```python
from build123d import *

# Parameters (mm, degrees)
F0_R      = 2
F1_DEPTH  = 6
F3_DEPTH  = 6.001
F5_DEPTH  = 6.001
F6_R      = 5
F7_DEPTH  = 6.001
F8_DEPTH  = 585
F9_R      = 2
F10_DEPTH = 6.001
F12_DEPTH = 2.5
F13_R     = 2


# Not quite as in the source:
# - an extrude ends at something that could not be found from the text; its depth is read off the source's solid


with BuildPart() as f1:
    # F0 (on Front) → F1 (new body)
    with BuildSketch(Plane.XZ):
        with BuildLine():
            Line((61.1081310213, 8.0650188029), (-54.7722764313, 8.0650188029))
            ThreePointArc((-54.7722764313, 8.0650188029), (-58.9525619371, 3.7295520634), (-59.8848706484, -2.2203940898))
            Line((-59.8848706484, -2.2203940898), (-59.8848706484, -29.6689261496))
            ThreePointArc((-59.8848706484, -29.6689261496), (-58.4204045543, -33.2044600555), (-54.8848706484, -34.6689261496))
            Line((-54.8848706484, -34.6689261496), (-38.6363018323, -34.6689261496))
            Line((-38.6363018323, -34.6689261496), (39.8797094822, -34.6689261496))
            Line((39.8797094822, -34.6689261496), (177.1196573973, -60.5151057243))
            Line((177.1196573973, -60.5151057243), (247.381187493, -88.5924363301))
            Line((247.381187493, -88.5924363301), (248.0585300922, -163.5853774846))
            Line((248.0585300922, -163.5853774846), (308.0585300922, -163.5853774846))
            Line((308.0585300922, -163.5853774846), (308.0585300922, -13.5853774846))
            Line((308.0585300922, -13.5853774846), (61.1081310213, 8.0650188029))
        make_face()
        with Locations((35.7915443742, -3.0683759738)):
            Circle(F0_R, mode=Mode.SUBTRACT)
    extrude(amount=F1_DEPTH)

    # F2 (on face) → F3 (cut, through all)
    with BuildSketch(Plane.XZ.offset(6)):
        with BuildLine():
            ThreePointArc((92.5020176823, -9.2679053605), (88.9664837764, -17.8034392664), (97.5020176823, -14.2679053605))
            ThreePointArc((97.5020176823, -14.2679053605), (96.0375515883, -10.7323714546), (92.5020176823, -9.2679053605))
        make_face()
    extrude(amount=-F3_DEPTH, mode=Mode.SUBTRACT)

    # F4 (on face) → F5 (cut, through all)
    with BuildSketch(Plane.XZ.offset(6)):
        with BuildLine():
            ThreePointArc((284.0794362254, -115.9942394993), (281.9581158818, -121.1155598429), (287.0794362254, -118.9942394993))
            ThreePointArc((287.0794362254, -118.9942394993), (286.2007565689, -116.8729191558), (284.0794362254, -115.9942394993))
        make_face()
        with BuildLine():
            ThreePointArc((287.0794362254, -56.0820794532), (281.9581158818, -53.9607591097), (284.0794362254, -59.0820794532))
            ThreePointArc((284.0794362254, -59.0820794532), (286.2007565689, -58.2033997968), (287.0794362254, -56.0820794532))
        make_face()
    extrude(amount=-F5_DEPTH, mode=Mode.SUBTRACT)

    # F6 (on face) → F7 (cut, through all)
    with BuildSketch(Plane(origin=(0, 0, 0), x_dir=(-1, 0, 0), z_dir=(0, 1, 0))):
        with Locations((7.8367077125, 0)):
            Circle(F6_R)
    extrude(amount=-F7_DEPTH, mode=Mode.SUBTRACT)

    # F0 (on Front) → F8 (cut, through all)
    with BuildSketch(Plane.XZ):
        with BuildLine():
            Line((61.1081310213, 8.0650188029), (-54.7722764313, 8.0650188029))
            ThreePointArc((-54.7722764313, 8.0650188029), (-58.9525619371, 3.7295520634), (-59.8848706484, -2.2203940898))
            Line((-59.8848706484, -2.2203940898), (-59.8848706484, -29.6689261496))
            ThreePointArc((-59.8848706484, -29.6689261496), (-58.4204045543, -33.2044600555), (-54.8848706484, -34.6689261496))
            Line((-54.8848706484, -34.6689261496), (-38.6363018323, -34.6689261496))
            Line((-38.6363018323, -34.6689261496), (39.8797094822, -34.6689261496))
            Line((39.8797094822, -34.6689261496), (177.1196573973, -60.5151057243))
            Line((177.1196573973, -60.5151057243), (247.381187493, -88.5924363301))
            Line((247.381187493, -88.5924363301), (248.0585300922, -163.5853774846))
            Line((248.0585300922, -163.5853774846), (308.0585300922, -163.5853774846))
            Line((308.0585300922, -163.5853774846), (308.0585300922, -13.5853774846))
            Line((308.0585300922, -13.5853774846), (61.1081310213, 8.0650188029))
        make_face()
        with Locations((35.7915443742, -3.0683759738)):
            Circle(F0_R, mode=Mode.SUBTRACT)
    extrude(amount=-F8_DEPTH, mode=Mode.SUBTRACT)

    # F9 (on face) → F10 (cut, through all)
    with BuildSketch(Plane.XZ.offset(6)):
        with Locations((144.0575271969, -19.352506299)):
            Circle(F9_R)
    extrude(amount=-F10_DEPTH, mode=Mode.SUBTRACT)

    # F11 (on face) → F12 (cut)
    with BuildSketch(Plane(origin=(0, 0, 0), x_dir=(-1, 0, 0), z_dir=(0, 1, 0))):
        Polygon((-95.3768665934, -0.9623710934), (-95.9008827898, 5.0147023565), (-298.1252011792, -12.7145122896), (-308.0585300922, -13.5853774846), (-308.0585300922, -19.6083919751), (-297.6011849827, -18.6915857396), align=None)
    extrude(amount=-F12_DEPTH, mode=Mode.SUBTRACT)

    # F13
    f13_edges = [f1.edges().sort_by_distance(p)[0] for p in [
        (308.05853, -4.25, -13.585377),
    ]]
    fillet(f13_edges, radius=F13_R)


solid = f1.part
```
Input: part model. Units: mm. Frame: model coordinates. A direction names the side the tool comes from. Round coordinates to 2 decimals unless told otherwise and drop trailing zeros. Order: outer loops, then holes, each group sorted by start corner. A loop starts at its lowest first (then second) coordinate and runs counter-clockwise, first axis right, second up. Notation, with made-up numbers: (58.5, 83) - (107.5, 83) arc R13 cw to (107.5, 108) - close; hole circle Ø6 at (-27, 54.25). An arc over 180 degrees is marked (long way). Answer in a Markdown table with one row per item.
Item 1: Mould query, pull axis X, two halves, no side actions, for faces 3 (the cylindrical face through (-2.84, -2.96, 0.22)), 4 (the flat face through (107.54, -2.96, -47.41)), 5 (the flat face through (164, 0, -46)), 6 (the flat face through (185.39, -4.29, -2.83)). Classes: released by +X, released by -X, zero draft, split by the parting line, or undercut.
Model answer:
| item | result |
|---|---|
| face 3 | undercut |
| face 4 | released by -X |
| face 5 | zero draft |
| face 6 | released by +X |
Item 2: Section query B-B (x = 254.5). Return the cut outline in (y, z).
Model answer:
| item | result |
|---|---|
| outline | (-6, -163.59) - (0, -163.59) - (0, -14.91) - (-2.5, -14.91) - (-2.5, -8.89) - (-6, -8.89) - close |
Item 3: Section query A-A (y = -1). Return the cut outline in (x, z), then the cut area to 3 significant figures.
Model answer:
| item | result |
|---|---|
| outline | (-59.88, -29.67) arc R5 ccw to (-54.88, -34.67) - (39.88, -34.67) - (177.12, -60.52) - (247.38, -88.59) - (248.06, -163.59) - (308.06, -163.59) - (308.06, -19.61) - (95.38, -0.96) - (95.9, 5.01) - (61.11, 8.07) - (-54.77, 8.07) arc R10 ccw to (-59.88, -2.22) - close; hole circle Ø10 at (-7.84, 0); hole circle Ø4 at (35.79, -3.07); hole circle Ø10 at (92.5, -14.27); hole circle Ø4 at (144.06, -19.35); hole circle Ø6 at (284.08, -118.99); hole circle Ø6 at (284.08, -56.08) |
| area | 23,900 mm² |
Item 4: Line query: line 1 (Z direction, x = 26, y = -4.2); line 2 (X direction, y = -4.6, z = -118); line 3 (X direction, y = -3.95, z = -15). Output: solid intervals per line, ascending.
Model answer:
| item | result |
|---|---|
| line 1 | z = -34.67 to 8.07 |
| line 2 | x = 247.65 to 281.25, 286.91 to 308.06 |
| line 3 | x = -59.88 to 87.56, 97.45 to 308.01 |
Item 5: Reachability of faces 1 (the flat face through (202, -2.5, -7)), 2 (the flat face through (164, -6, -52)) from +Z, -Z, +X, -X, +Y, -Y: full face, straight path, thin tool, end or side. Return the list, or none.
Model answer:
| item | result |
|---|---|
| face 1 | +Z, +X, +Y |
| face 2 | +Z, -Z, +X, -X, -Y |
Item 6: Pin query (flat end, axial travel): pin 1 (3 mm diameter, centred on x = 16, y = -1.5, fed in from -Z); pin 2 (3.5 mm diameter, centred on x = 35.79, z = -3.07, fed in from -Y); pin 3 (3 mm diameter, centred on x = 96.5, y = -5, fed in from +Z). Return the tip coordinate at first contact, or that it passes through.
Model answer:
| item | result |
|---|---|
| pin 1 | stops at z = -34.67 |
| pin 2 | passes through |
| pin 3 | stops at z = 5.09 |
Item 7: Section query C-C (z = -98). Return the cut outline in (x, y), then the cut area to 3 significant figures.
Model answer:
| item | result |
|---|---|
| outline | (247.47, -6) - (308.06, -6) - (308.06, 0) - (247.47, 0) - close |
| area | 364 mm² |
Item 8: Section query D-D (z = -67). Return the cut outline in (x, y), then the cut area to 3 significant figures.
Model answer:
| item | result |
|---|---|
| outline | (193.35, -6) - (308.06, -6) - (308.06, 0) - (193.35, 0) - close |
| area | 688 mm² |
